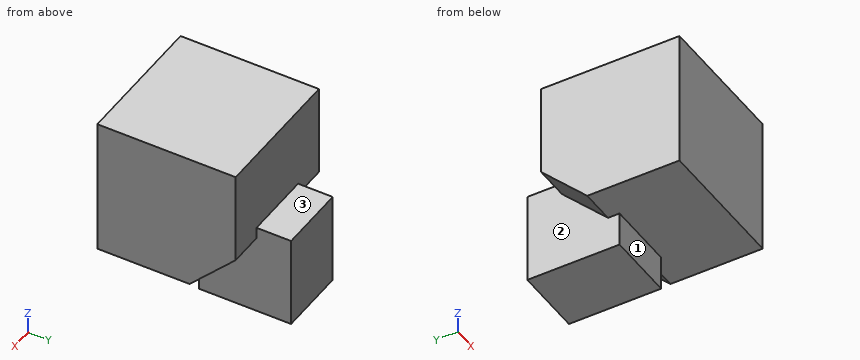
```python
from build123d import *

# Parameters (mm, degrees)
F0_W     = 19.05
F0_H     = 19.05
F1_DEPTH = 19.05
F4_DEPTH = 19.05
F5_W     = 12.7
F5_H     = 12.7
F6_DEPTH = 4.7625


with BuildPart() as f1:
    # F0 (on Front) → F1 (new body)
    with BuildSketch(Plane.XZ):
        with Locations((9.525, 9.525)):
            Rectangle(F0_W, F0_H)
    extrude(amount=-F1_DEPTH)

    # F3 (on face) → F4 (cut)
    with BuildSketch(Plane.YZ.offset(19.05)):
        Polygon((19.05, 6.35), (12.7, 0), (19.05, 0), align=None)
    extrude(amount=-F4_DEPTH, mode=Mode.SUBTRACT)

    # F5 (on offset) → F6 (join, symmetric)
    with BuildSketch(Plane.YZ.offset(9.525)):
        with Locations((17.4625, 1.5875)):
            Rectangle(F5_W, F5_H)
    extrude(amount=F6_DEPTH, both=True)


solid = f1.part
```
Can you work these out from the model? Positions are in its coordinate system, mm. Face numbers are marked on the shaded views. A direction names the side the tool comes from. Round coordinates to 2 decimals unless told otherwise and drop trailing zeros. Loops run counter-clockwise (first coordinate to the right, second up) from the corner with the lowest first, then second, coordinate; pieces in that order, holes last. Notation, with made-up numbers: M 32,3.25 L 37,3.25 A19 cw 37,21.25 Z; hole C 13,20 d10. An arc over 180 degrees is marked long. Write item = value, one per line. Start each with the question number.
(1) Suppose I cut it at C-C on x = 18. Write out the boundary of the cut face in (y, z).
(2) Suppose I cut it at B-B on z = 4.25. Write out the boundary of the cut face in (x, y).
(3) Suppose I cut it at D-D on z = 17. Write out the boundary of the cut face in (x, y), plus the area to 3 significant figures.
(4) I'm going to push flat-ended pins straight in: P1, Ø5, axis at x = 9.5, y = 22.5, coming from the +Z side; P2, Ø3, axis at x = 6, z = 14.5, coming from the +Y side; P3, Ø4, axis at x = 6, y = 7.5, coming from the -Z side. Where does each tip first touch, or does it pass through?
(5) Which directions (+Z, -Z, +X, -X, +Y, -Y) give clear straight access to the entire face, cutting with the end or side of a thin tool? Please do the marked faces 1, 2 and 3.
(6) Suppose I cut it at A-A on y = 13.5. Write out the boundary of the cut face in (x, z).
(7) I need wall thicknesses on line 1 along Y through (x, z) = (14, 17.75); line 2 along Y through (x, z) = (13, -0.5). Which ranges of each line are inside material? Lowest first, please.
Answer block:
q1.outline = M 0,0 L 12.7,0 L 19.05,6.35 L 19.05,19.05 L 0,19.05 Z
q2.outline = M 0,0 L 19.05,0 L 19.05,16.95 L 14.29,16.95 L 14.29,23.81 L 4.76,23.81 L 4.76,16.95 L 0,16.95 Z
q3.outline = M 0,0 L 19.05,0 L 19.05,19.05 L 0,19.05 Z
q3.area = 363 mm²
q4.P1 = 7.94
q4.P2 = 19.05
q4.P3 = 0
q5.face_1 = -Z, +X, -X, -Y
q5.face_2 = -Z, -X, +Y
q5.face_3 = +Z, +X, -X, +Y
q6.outline = M 0,0.8 L 4.76,0.8 L 4.76,-4.76 L 14.29,-4.76 L 14.29,0.8 L 19.05,0.8 L 19.05,19.05 L 0,19.05 Z
q7.line_1 = 0 to 19.05
q7.line_2 = 11.11 to 23.81
